The drawing under review shows one solid part. Ordinate dimensions are in mm from its lowest x, y, z. Give positions to 0.01 mm unless a question says otherwise; leave off trailing zeros. Loops run counter-clockwise (first coordinate to the right, second up) from the corner with the lowest first, then second, coordinate; pieces in that order, holes last.
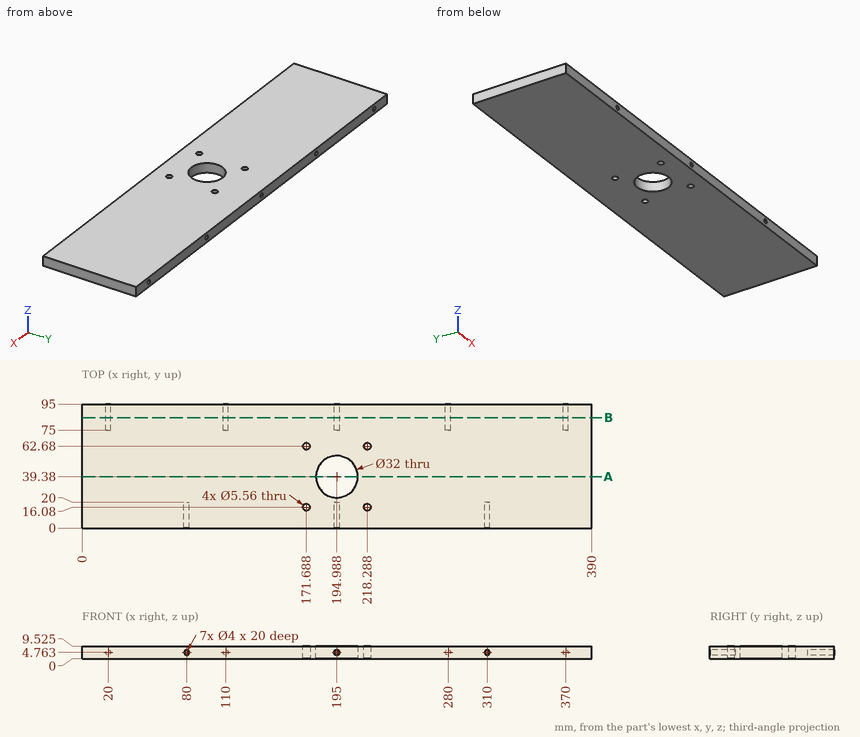
Item 1: Take a section at A-A on y = 39.38. Give the boundary of the cut face in (x, z) (1 decimal).
Answer:
outline: (0, 0) - (179, 0) - (179, 9.5) - (0, 9.5) - close; (211, 0) - (390, 0) - (390, 9.5) - (211, 9.5) - close
Item 2: Clearance check with a flat-ended pin moving along its axis: pin 1 Ø2 at (x, z) = (280.5, 4.5) entering from +Y. State where the tip first meets the part, or that it passes through.
Answer:
pin 1: stops at y = 75
Item 3: Take a section at B-B on y = 84.5. Give the boundary of the cut face in (x, z) (1 decimal), and give its area (3 significant figures).
Answer:
outline: (0, 0) - (390, 0) - (390, 9.5) - (0, 9.5) - close; hole circle Ø4 at (20, 4.8); hole circle Ø4 at (110, 4.8); hole circle Ø4 at (195, 4.8); hole circle Ø4 at (280, 4.8); hole circle Ø4 at (370, 4.8)
area: 3,650 mm2
Item 4: For L1, parallel to X at y = 12, z = 5 (1 decimal); L2, parallel to Z at x = 20, y = 86 (1 decimal); L3, parallel to X at y = 40, z = 3 (1 decimal), list the stretches that pass through material, from the lowest coordinate up.
Answer:
L1: x = 0 to 78, 82 to 193, 197 to 308, 312 to 390
L2: z = 0 to 2.8, 6.8 to 9.5
L3: x = 0 to 179, 211 to 390
